The model under review builds one solid part; all positions refer to its coordinate system, in mm. Face numbers are marked on the shaded views. Give positions to 0.01 mm unless a question says otherwise; leave off trailing zeros. Write each loop counter-clockwise with the first axis right and the second up, starting at its lowest first coordinate (ties: lowest second). Pieces come first, ordered by that corner, then holes.
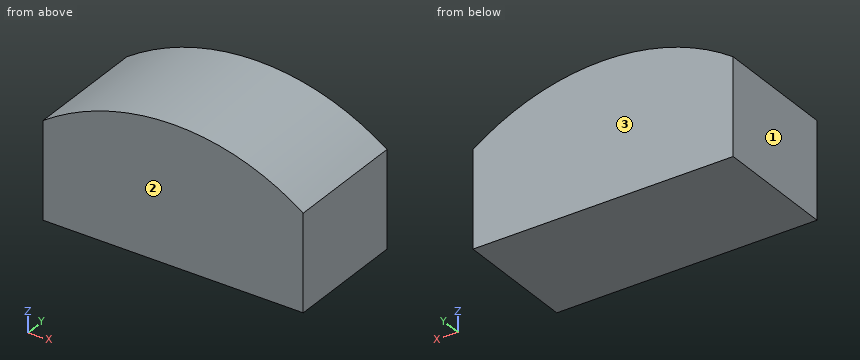
from build123d import *

# Parameters (mm, degrees)
EXTRUDE_START            = -329.393398282
EXTRUDE_1_DEPTH          = 367.123106012
CUT_EXTRUDE_2_REACH      = 654.668
CUT_EXTRUDE_2_END_RADIUS = 675
SKETCH_4_W               = 770
SKETCH_4_H               = 357.123106012


# Read off the part's stored shape, not the designer's step: 凸台-拉伸1
with BuildPart() as part:
    # 凸台-拉伸1 outline → 凸台-拉伸1 (new body)
    with BuildSketch(Plane(origin=(0, 0, 0), x_dir=(1, 0, 0), z_dir=(0, 1, 0)).offset(EXTRUDE_START)):
        with BuildLine():
            Line((390, -288.70946964), (390, 0))
            Line((390, 0), (-390, 0))
            Line((-390, 0), (-390, -288.70946964))
            ThreePointArc((-390, -288.70946964), (0, -411.663690552), (390, -288.70946964))
        make_face()
    extrude(amount=EXTRUDE_1_DEPTH)

    # 切除-拉伸2: up to this cylinder (the profile starts inside it)
    cut_extrude_2_end = Plane(origin=(0, -145.831845, -268.336309448), z_dir=(0, 1, 0)) * Cylinder(CUT_EXTRUDE_2_END_RADIUS, 2660.336, mode=Mode.PRIVATE)
    # 草图4 → 切除-拉伸2 (cut, up to the surface)
    with BuildSketch(Plane(origin=(0, 0, 5), x_dir=(-1, 0, 0), z_dir=(0, 0, -1)), mode=Mode.PRIVATE) as cut_extrude_2_sk1:
        with Locations((0, -145.831845276)):
            Rectangle(SKETCH_4_W, SKETCH_4_H)
    cut_extrude_2_tool1 = extrude(cut_extrude_2_sk1.sketch, amount=-CUT_EXTRUDE_2_REACH, mode=Mode.PRIVATE) & cut_extrude_2_end
    add(cut_extrude_2_tool1.solids().sort_by_distance((0, -145.831845, 5))[0], mode=Mode.SUBTRACT)


solid = part.part
1) Consider section A-A, the plane y = 4. Give the boundary of the cut face in (x, z), then the cut area to 3 significant figures.
2) To check wall thickness, follow probe 1 along X at (y, z) = (-273, 27.5); probe 2 along Y at (x, z) = (117, 268); probe 3 along Z at (x, y) = (228, -277). State the ranges of each line that lie inside material, in increasing order.
3) The part is to be moulded in two halves that separate along Y. For the marked faces 1, 2 and 3, say which applies: +Y half, -Y half, draft (parallel to the pull), parting line (faces both ways), or undercut.
4) Consider section B-B, the plane z = 191. Give the boundary of the cut face in (x, y).
5) Insertion check: pin 1 (8 mm diameter, centred on x = 244, y = -252.5, fed in from +Z); pin 2 (10 mm diameter, centred on x = -172, y = -69.5, fed in from +Z). Each pin has a flat end and moves straight along its axis. Give the tip position at first contact, or say it passes through.
Answer block:
1. outline: (-390, 0) - (390, 0) - (390, 288.71) arc R680 ccw to (-390, 288.71) - close; hole (-385, 5) - (385, 5) - (385, 286.1) arc R675 ccw to (-385, 286.1) - close
1. area: 10,800 mm2
2. probe 1: x = -390 to -385, 385 to 390
2. probe 2: y = -329.39 to -324.39, 32.73 to 37.73
2. probe 3: z = 0 to 5, 366.99 to 372.3
3. face 1: draft
3. face 2: -Y half
3. face 3: +Y half
4. outline: (-390, -329.39) - (390, -329.39) - (390, 37.73) - (-390, 37.73) - close; hole (-385, -324.39) - (385, -324.39) - (385, 32.73) - (-385, 32.73) - close
5. pin 1: stops at z = 367.9
5. pin 2: stops at z = 390.84
